Input: part model. Units: mm. Frame: model coordinates. A direction names the side the tool comes from. Coordinates: 2 decimals unless noted, no trailing zeros. Loops run counter-clockwise (first coordinate to the right, second up) from the corner with the lowest first, then second, coordinate; pieces in that order, holes last. Notation, with made-up numbers: (-5, 69.5) - (23, 69.5) arc R19 cw to (23, 89.5) - close; hole circle Ø9 at (35.5, -13). An arc over 180 degrees is marked (long way). Use a Markdown table: item, result. Add a question column.
1. Section query D-D on x = 0. Return the cut outline in (y, z), then the cut area to 3 significant figures.
2. Contact query for flat-ended pins moving along their axis: P1, Ø5.5, axis at x = 57, y = 19.5, coming from the +Z side; P2, Ø9, axis at x = 59.5, y = -18, coming from the +Z side; P3, Ø5.5, axis at x = 58, y = -18, coming from the +Z side. Output: stop coordinate, or through.
3. Section query B-B on x = 58. Return the cut outline in (y, z).
4. Section query A-A on y = -18. Return the cut outline in (x, z), then the cut area to 3 significant figures.
5. Ray query, L1, parallel to Y at x = 58, z = 1.7; L2, parallel to Y at x = 0, z = 6.75; L3, parallel to Z at x = -62.5, y = 22. Return the intervals inside material, ascending. Write a range as [from, to].
6. Draft query along X for faces 1 (the face through (-70, 0, 5)), 2 (the face through (70, 0, 5)), 3 (the face through (52.505, 19.242, 6.845)). Return one class per face: released by +X, released by -X, zero draft, split by the parting line, or undercut.
7. Section query C-C on z = 6.5. Return the cut outline in (x, y).
8. Access query for faces 4 (the face through (-54.7, -17.9, 1.8)), 5 (the face through (-58, 15, 3.6)). Directions: +Z, -Z, +X, -X, +Y, -Y. A direction counts if a zero-diameter tool reaches every point of the face in a straight line with its end or side. Return the directions, or none.
```python
from build123d import *

# Parameters (mm, degrees)
SKETCH1_W                                           = 140
SKETCH1_H                                           = 56
EXTRUDE1_DEPTH                                      = 10
CBORE_FOR_M6_HEX_SOCKET_HEAD_CAP_SCREW1_D           = 6.6
CBORE_FOR_M6_HEX_SOCKET_HEAD_CAP_SCREW1_CBORE_D     = 11
CBORE_FOR_M6_HEX_SOCKET_HEAD_CAP_SCREW1_CBORE_DEPTH = 6.4


with BuildPart() as part:
    # Sketch1 → Extrude1 (new body)
    with BuildSketch(Plane.XY):
        Rectangle(SKETCH1_W, SKETCH1_H)
    extrude(amount=EXTRUDE1_DEPTH)

    # CBORE for M6 Hex Socket Head Cap Screw1 (through all)
    with Locations(Plane.XY.offset(10)):
        with Locations((58, -18), (58, 19), (0, -18), (-58, -18), (-58, 19)):
            CounterBoreHole(CBORE_FOR_M6_HEX_SOCKET_HEAD_CAP_SCREW1_D / 2, CBORE_FOR_M6_HEX_SOCKET_HEAD_CAP_SCREW1_CBORE_D / 2, CBORE_FOR_M6_HEX_SOCKET_HEAD_CAP_SCREW1_CBORE_DEPTH)


solid = part.part
```
Resolved:
| question | item | result |
|---|---|---|
| 1 | outline | (-28, 0) - (-21.3, 0) - (-21.3, 3.6) - (-23.5, 3.6) - (-23.5, 10) - (-28, 10) - close; (-14.7, 0) - (28, 0) - (28, 10) - (-12.5, 10) - (-12.5, 3.6) - (-14.7, 3.6) - close |
| 1 | area | 466 mm² |
| 2 | P1 | z = 3.6 |
| 2 | P2 | z = 10 |
| 2 | P3 | through |
| 3 | outline | (-28, 0) - (-21.3, 0) - (-21.3, 3.6) - (-23.5, 3.6) - (-23.5, 10) - (-28, 10) - close; (-14.7, 0) - (15.7, 0) - (15.7, 3.6) - (13.5, 3.6) - (13.5, 10) - (-12.5, 10) - (-12.5, 3.6) - (-14.7, 3.6) - close; (22.3, 0) - (28, 0) - (28, 10) - (24.5, 10) - (24.5, 3.6) - (22.3, 3.6) - close |
| 4 | outline | (-70, 0) - (-61.3, 0) - (-61.3, 3.6) - (-63.5, 3.6) - (-63.5, 10) - (-70, 10) - close; (-54.7, 0) - (-3.3, 0) - (-3.3, 3.6) - (-5.5, 3.6) - (-5.5, 10) - (-52.5, 10) - (-52.5, 3.6) - (-54.7, 3.6) - close; (3.3, 0) - (54.7, 0) - (54.7, 3.6) - (52.5, 3.6) - (52.5, 10) - (5.5, 10) - (5.5, 3.6) - (3.3, 3.6) - close; (61.3, 0) - (70, 0) - (70, 10) - (63.5, 10) - (63.5, 3.6) - (61.3, 3.6) - close |
| 4 | area | 1,120 mm² |
| 5 | L1 | [-28, -21.3], [-14.7, 15.7], [22.3, 28] |
| 5 | L2 | [-28, -23.5], [-12.5, 28] |
| 5 | L3 | [0, 3.6] |
| 6 | face 1 | released by -X |
| 6 | face 2 | released by +X |
| 6 | face 3 | undercut |
| 7 | outline | (-70, -28) - (70, -28) - (70, 28) - (-70, 28) - close; hole circle Ø11 at (-58, -18); hole circle Ø11 at (-58, 19); hole circle Ø11 at (0, -18); hole circle Ø11 at (58, -18); hole circle Ø11 at (58, 19) |
| 8 | face 4 | +Z, -Z |
| 8 | face 5 | +Z |
